For this review, take the finished solid that the model builds, in its own axes (mm). A direction names the side the tool comes from. Give positions to 0.01 mm unless a question says otherwise; leave off trailing zeros. Write each loop counter-clockwise with the first axis right and the second up, starting at its lowest first coordinate (ties: lowest second). Pieces come first, ordered by that corner, then holes. Notation, with made-up numbers: M -19.5,33 L 31.5,33 A20 ccw 31.5,40 Z; hole C 77.25,86.5 d3. An arc over 180 degrees is marked long. One line per item, written item: value. Start each with the question number.
Item 1: Consider section B-B, the plane x = 10. Write out the cut boundary in (y, z), and give its area (3 significant figures).
Item 2: To check wall thickness, follow probe 1 along Z at (x, y) = (0, -14); probe 2 along Z at (x, y) = (4.5, -4.5); probe 3 along X at (y, z) = (2, 34). State the ranges of each line that lie inside material, in increasing order.
Item 3: Mouldability with a two-part tool opening along X and no side actions: class faces 3 (the face through (-20, -3, 23)), 4 (the face through (-0.37, -12.54, 28.34)), 5 (the face through (0, -5, 10)) as released by +X, released by -X, zero draft, split by the parting line, or undercut.
Item 4: Consider section D-D, the plane y = 3.75. Write out the cut boundary in (x, z).
Item 5: Consider section A-A, the plane y = -6.75. Write out the cut boundary in (x, z), and give its area (3 significant figures).
Item 6: Tool access review of faces 1 (the face through (19, -10, 2)), 2 (the face through (0, 3, 36.25)): name each direction out of +Z, -Z, +X, -X, +Y, -Y from which nothing blocks a thin tool from reaching the whole face with its end or side.
Item 7: Consider section C-C, the plane z = 30. Write out the cut boundary in (x, y).
Item 8: Clearance check with flat-ended pins moving along their axes: pin 1 Ø2 at (x, y) = (-12, 6) entering from -Z; pin 2 Ø4.5 at (x, z) = (0, 30) entering from +Y; pin 3 Ø2 at (x, z) = (15.5, 16) entering from +Y. State where each tip first meets the part, or that it passes through.
```python
from build123d import *

# Parameters (mm, degrees)
F0_W     = 40
F0_H     = 20
F0_H_2   = 10
F1_DEPTH = 40
F2_DEPTH = 20
F3_R     = 2.15
F3_R_2   = 1.7
F4_DEPTH = 40
F5_W     = 12.5
F5_H     = 12.5
F5_R     = 1.7
F6_DEPTH = 25
F7_R     = 5


with BuildPart() as f1:
    # F0 (on Top) → F1 (new body)
    with BuildSketch(Plane.XY):
        with Locations((0, 5)):
            Rectangle(F0_W, F0_H)
        with Locations((0, -10)):
            Rectangle(F0_W, F0_H_2)
    extrude(amount=F1_DEPTH)

    # F0 (on Top) → F2 (cut)
    with BuildSketch(Plane.XY):
        with Locations((0, 5)):
            Rectangle(F0_W, F0_H)
    extrude(amount=F2_DEPTH, mode=Mode.SUBTRACT)

    # F3 (on face) → F4 (cut)
    with BuildSketch(Plane.XZ.offset(15)):
        with Locations((-10, 10)):
            Circle(F3_R)
        with Locations((10, 10)):
            Circle(F3_R)
        with Locations((0, 30)):
            Circle(F3_R_2)
    extrude(amount=-F4_DEPTH, mode=Mode.SUBTRACT)

    # F5 (on face) → F6 (cut)
    with BuildSketch(Plane(origin=(0, 15, 0), x_dir=(-1, 0, 0), z_dir=(0, 1, 0))):
        with Locations((0, 30)):
            Rectangle(F5_W, F5_H)
        with Locations((0, 30)):
            Circle(F5_R, mode=Mode.SUBTRACT)
    extrude(amount=-F6_DEPTH, mode=Mode.SUBTRACT)

    # F7
    f7_edges = [f1.edges().sort_by_distance(p)[0] for p in [
        (-20, -10, 0),
        (20, -10, 0),
        (-20, 0, 40),
        (20, 0, 40),
    ]]
    fillet(f7_edges, radius=F7_R)


solid = f1.part
```
Model answer:
1. outline: M -15,0 L -5,0 L -5,7.85 L -15,7.85 Z; M -15,12.15 L -5,12.15 L -5,20 L 15,20 L 15,40 L -15,40 Z
1. area: 757 mm2
2. probe 1: z = 0 to 28.3, 31.7 to 40
2. probe 2: z = 20 to 23.75, 36.25 to 40
2. probe 3: x = -20 to -6.25, 6.25 to 20
3. face 3: released by -X
3. face 4: undercut
3. face 5: zero draft
4. outline: M -20,20 L 20,20 L 20,35 A5 ccw 15,40 L -15,40 A5 ccw -20,35 Z; hole M -6.25,23.75 L 6.25,23.75 L 6.25,36.25 L -6.25,36.25 Z
5. outline: M -20,5 A5 ccw -15,0 L 15,0 A5 ccw 20,5 L 20,35 A5 ccw 15,40 L -15,40 A5 ccw -20,35 Z; hole C -10,10 d4.3; hole M -6.25,23.75 L 6.25,23.75 L 6.25,36.25 L -6.25,36.25 Z; hole C 10,10 d4.3
5. area: 1,390 mm2
6. face 1: -Z, +X, +Y, -Y
6. face 2: +Y
7. outline: M -20,-15 L -1.7,-15 L -1.7,-10 L -6.25,-10 L -6.25,15 L -20,15 Z; M 1.7,-15 L 20,-15 L 20,15 L 6.25,15 L 6.25,-10 L 1.7,-10 Z
8. pin 1: stops at z = 20
8. pin 2: stops at y = -10
8. pin 3: stops at y = -5
